Check sheet for the modelled part. Datum: model origin and axes. Units: mm. Give positions to 0.01 mm unless a question says otherwise; leave off trailing zeros. Write each loop counter-clockwise with the first axis right and the second up, starting at its lowest first coordinate (ties: lowest second). Pieces come first, ordered by that corner, then holes.
from build123d import *

# Parameters (mm, degrees)
F0_R     = 100
F0_R_2   = 2.25
F0_R_3   = 16
F1_DEPTH = 1
F4_SIZE  = 0.5


with BuildPart() as f1:
    # F0 (on Top) → F1 (new body, symmetric)
    with BuildSketch(Plane.XY):
        Circle(F0_R)
        with Locations((0, -20)):
            Circle(F0_R_2, mode=Mode.SUBTRACT)
        Circle(F0_R_3, mode=Mode.SUBTRACT)
    extrude(amount=F1_DEPTH, both=True)

    # F2 (on Right) → F3 (revolve, cut)
    with BuildSketch(Plane.YZ):
        Polygon((-100, 1.035245), (-100, 0), (-99.477045, 0.301928), (-92.5, 1.035245), align=None)
        Polygon((-99.477045, -0.301928), (-100, 0), (-100, -1.035245), (-92.5, -1.035245), align=None)
    revolve(axis=Axis((0, 0, 4.501528), (0, 0, 1)), mode=Mode.SUBTRACT)

    # F4
    f4_edges = [f1.edges().sort_by_distance(p)[0] for p in [
        (-16, 0, 1),
        (-16, 0, -1),
        (-2.25, -20, 1),
        (-2.25, -20, -1),
    ]]
    chamfer(f4_edges, length=F4_SIZE)


solid = f1.part
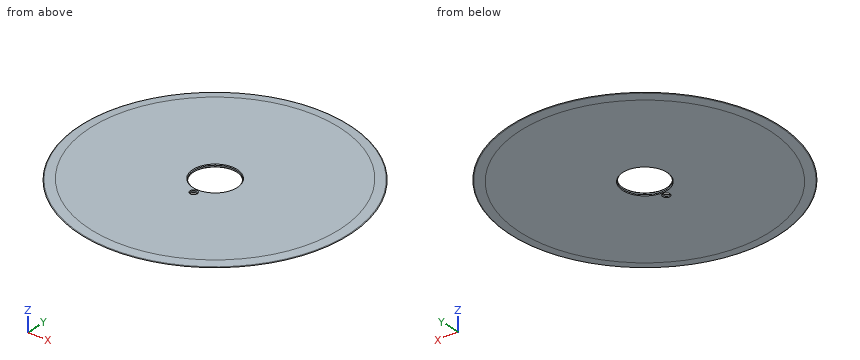
1) Sectioned sample at A-A on y = 0. Record the boundary of the cut face in (x, z).
2) Gauge pin test, flat end, axial feed: pin 1 (5 mm diameter, centred on x = 0, y = -20, fed in from -Z). Record the tip position at first contact, or that the pin passes through.
3) Scan lines: L1, parallel to Z at x = -57.5, y = -73; L2, parallel to Y at x = 11, z = 0.15; L3, parallel to X at y = 71, z = -0.1. Record each from-to range of solid material in increasing order.
Answers below:
1. outline: (-100, 0) - (-99.48, -0.3) - (-92.84, -1) - (-16.5, -1) - (-16, -0.5) - (-16, 0.5) - (-16.5, 1) - (-92.84, 1) - (-99.48, 0.3) - close; (16, -0.5) - (16.5, -1) - (92.84, -1) - (99.48, -0.3) - (100, 0) - (99.48, 0.3) - (92.84, 1) - (16.5, 1) - (16, 0.5) - close
2. pin 1: stops at z = -0.75
3. L1: z = -0.99 to 0.99
3. L2: y = -99.13 to -11.62, 11.62 to 99.13
3. L3: x = -70.17 to 70.17
